from build123d import *
from OCP.BRepFilletAPI import BRepFilletAPI_MakeChamfer

# Parameters (mm, degrees)
BOSS_EXTRUDE1_DEPTH = 50
BOSS_EXTRUDE2_DEPTH = 100
SKETCH3_R           = 25
CUT_EXTRUDE1_DEPTH  = 1015.958328012
FILLET1_R           = 10
CHAMFER1_SIZE       = 40
CHAMFER1_SIZE2      = 23.094010768


with BuildPart() as part:
    # Sketch1 → Boss-Extrude1 (new body)
    with BuildSketch(Plane.XY):
        Polygon((0, 0), (592.5, 0), (643.63, 88.559757791), (-643.63, 88.559757791), (-592.5, 0), align=None)
    extrude(amount=BOSS_EXTRUDE1_DEPTH)

    # Sketch2 → Boss-Extrude2 (add)
    with BuildSketch(Plane(origin=(0, 0, 0), x_dir=(-1, 0, 0), z_dir=(0, 0, -1))):
        Polygon((-312.5, 0), (-262.5, 0), (-262.5, 88.559757791), (-362.5, 88.559757791), (-362.5, 0), align=None)
        Polygon((262.5, 88.559757791), (262.5, 0), (312.5, 0), (362.5, 0), (362.5, 88.559757791), align=None)
    extrude(amount=BOSS_EXTRUDE2_DEPTH)

    # Sketch3 → Cut-Extrude1 (cut, through all)
    with BuildSketch(Plane(origin=(362.5, 0, 0), x_dir=(0, 0, -1), z_dir=(1, 0, 0))):
        with Locations((50, 44.279878895)):
            Circle(SKETCH3_R)
    extrude(amount=-CUT_EXTRUDE1_DEPTH, mode=Mode.SUBTRACT)

    # Fillet1
    fillet1_edges = [part.edges().sort_by_distance(p)[0] for p in [
        (-312.5, 88.559757791, -100),
        (-312.5, 0, -100),
        (312.5, 88.559757791, -100),
        (312.5, 0, -100),
    ]]
    fillet(fillet1_edges, radius=FILLET1_R)

    # Chamfer1: one chamfer whose edges measure the first distance from different faces: ONE call of the kernel's chamfer builder (chamfer() names one face for all edges)
    chamfer1_edges_1 = [part.edges().sort_by_distance(p)[0] for p in [
        (-503.065, 88.559757791, 0),
    ]]
    chamfer1_side_1 = [part.faces().sort_by_distance(p)[0] for p in [
        (-490.708725047, 45.75636577, 0),
    ]]
    chamfer1_edges_2 = [part.edges().sort_by_distance(p)[0] for p in [
        (503.065, 88.559757791, 0),
    ]]
    chamfer1_side_2 = [part.faces().sort_by_distance(p)[0] for p in [
        (490.708725047, 45.75636577, 0),
    ]]
    chamfer1 = BRepFilletAPI_MakeChamfer(part.part.solid().wrapped)
    for e in chamfer1_edges_1:
        chamfer1.Add(CHAMFER1_SIZE, CHAMFER1_SIZE2, e.wrapped, chamfer1_side_1[0].wrapped)  # the first distance lies on this face
    for e in chamfer1_edges_2:
        chamfer1.Add(CHAMFER1_SIZE, CHAMFER1_SIZE2, e.wrapped, chamfer1_side_2[0].wrapped)  # the first distance lies on this face
    add(Compound.cast(chamfer1.Shape()), mode=Mode.REPLACE)


solid = part.part
Build history of the part. All positions in model axes, mm. A direction names the side the tool comes from. Round coordinates to 2 decimals unless told otherwise and drop trailing zeros. Write each loop counter-clockwise with the first axis right and the second up, starting at its lowest first coordinate (ties: lowest second). Pieces come first, ordered by that corner, then holes. Notation, with made-up numbers: (-23.75, -28.75) -> (9.25, -28.75) arc R25 cw to (9.25, -3.75) -> close; hole circle Ø11 at (45, 1). An arc over 180 degrees is marked (long way). Write item = value, one per line.
(1) Band-saw the part on B-B (x = 435). Give the cut face in (y, z).
Answer:
outline = (0, 0) -> (48.56, 0) -> (88.56, 23.09) -> (88.56, 50) -> (0, 50) -> close
(2) Two-plate mould, pull along Y, no slides. Class faces 5 (the face through (9, 88.56, 10)), 6 (the face through (313, 45, -100)), 7 (the face through (-311.8, 19.874, -44.58)): pulls with the +Y half, pulls with the -Y half, needs draft (parallel to the pull), parting line crosses it, or undercut.
Answer:
face_5 = pulls with the +Y half
face_6 = needs draft
face_7 = undercut
(3) Probe L1, parallel to Y at x = 332, z = -50; L2, parallel to X at y = 45.5, z = -18; L3, parallel to Z at x = -140, y = 45.5. List the from-to ranges inside material, lowest first.
Answer:
L1 = 0 to 19.28, 69.28 to 88.56
L2 = -362.5 to -262.5, 262.5 to 362.5
L3 = 0 to 50
(4) Flat gauge pins, fed straight in: pin 1 (2 mm diameter, centred on y = 73.5, z = -56, fed in from +X); pin 2 (24.5 mm diameter, centred on x = 457, y = 22.5, fed in from -Z); pin 3 (2 mm diameter, centred on y = 10, z = -57.5, fed in from -X); pin 4 (12 mm diameter, centred on x = 348.5, z = 20, fed in from -Y). Where does each tip first touch, or does it go through?
Answer:
pin_1 = 362.5
pin_2 = 0
pin_3 = -362.5
pin_4 = 0
(5) Band-saw the part on A-A (z = -13). Give the cut face in (x, y), then the cut area to 3 significant figures.
Answer:
outline = (-362.5, 0) -> (-262.5, 0) -> (-262.5, 88.56) -> (-362.5, 88.56) -> close; (262.5, 0) -> (362.5, 0) -> (362.5, 88.56) -> (262.5, 88.56) -> close
area = 17,700 mm2
(6) Band-saw the part on C-C (z = -63.5). Give the cut face in (x, y).
Answer:
outline = (-362.5, 0) -> (-262.5, 0) -> (-262.5, 23.24) -> (-362.5, 23.24) -> close; (-362.5, 65.32) -> (-262.5, 65.32) -> (-262.5, 88.56) -> (-362.5, 88.56) -> close; (262.5, 0) -> (362.5, 0) -> (362.5, 23.24) -> (262.5, 23.24) -> close; (262.5, 65.32) -> (362.5, 65.32) -> (362.5, 88.56) -> (262.5, 88.56) -> close
(7) Tool access for faces 1 (the face through (-493, 25, 0)), 2 (the face through (505.03, 68.84, 11.71)), 3 (the face through (-4, 45, 0)), 4 (the face through (-501.1, 68.84, 11.71)): list every direction of +Z, -Z, +X, -X, +Y, -Y with a clear straight run to the whole face (end or side of a thin tool).
Answer:
face_1 = -Z, -X, +Y, -Y
face_2 = -Z, +X, +Y
face_3 = -Z, +Y, -Y
face_4 = -Z, -X, +Y
(8) Band-saw the part on D-D (x = 6.5). Give the cut face in (y, z), then the cut area to 3 significant figures.
Answer:
outline = (0, 0) -> (88.56, 0) -> (88.56, 50) -> (0, 50) -> close
area = 4,430 mm2
